Model file for the job. Use its own axes, mm. Round coordinates to 2 decimals unless told otherwise and drop trailing zeros. Order: outer loops, then holes, each group sorted by start corner. A loop starts at its lowest first (then second) coordinate and runs counter-clockwise, first axis right, second up. Notation, with made-up numbers: (51.25, -18.75) -> (81.25, -18.75) arc R30 cw to (81.25, 8.25) -> close; hole circle Ø7 at (-28.5, 0.25). An arc over 180 degrees is marked (long way). Put each result on its own line as item: value. Start each with the question number.
Q1. Cut at A-A, the plane x = 164.5. List the corners of the cut face in (y, z).
Q2. Cut at C-C, the plane y = 25. List the corners of the cut face in (x, z), and give its area (3 significant figures).
Q3. Pull direction Y, two halves, no side cores. Call faces 1 (the face through (162.502, 4.588, 150.493)), 2 (the face through (86, 68, 148)): released by +Y, released by -Y, zero draft, split by the parting line, or undercut.
Q4. Flat gauge pins, fed straight in: P1, Ø1.6, axis at x = 103.5, z = 148.5, coming from the +Y side; P2, Ø0.6, axis at x = 6, z = 149, coming from the -Y side; P3, Ø5, axis at x = 164.5, y = 129.5, coming from the -Z side. Where does each tip first touch, or does it go through?
Q5. Cut at D-D, the plane z = 149.2. List the corners of the cut face in (x, y).
Q6. Probe L1, parallel to Y at x = 164.5, z = 150.45; L2, parallel to X at y = 129.5, z = 150.7; L3, parallel to Y at x = 163, z = 150.4. List the from-to ranges inside material, lowest first.
Q7. Cut at B-B, the plane y = 4.5. List the corners of the cut face in (x, z), and give its area (3 significant figures).
from build123d import *

# Parameters (mm, degrees)
SKETCH008_W     = 175
SKETCH008_H     = 140
PAD002_DEPTH    = 3
PAD003_DEPTH    = 2
SKETCH010_R     = 2
POCKET006_DEPTH = 3.001
CHAMFER001_SIZE = 2
FILLET001_R     = 3


with BuildPart() as part:
    # Sketch008 → Pad002 (new body)
    with BuildSketch(Plane.XY):
        with Locations((84.5, 67)):
            Rectangle(SKETCH008_W, SKETCH008_H)
    extrude(amount=PAD002_DEPTH)

    # Sketch009 → Pad003 (join)
    with BuildSketch(Plane.XY):
        Polygon((0.5, 9.5), (0.5, 124.5), (9.5, 124.5), (9.5, 133.5), (159.5, 133.5), (159.5, 124.5), (168.5, 124.5), (168.5, 9.5), (159.5, 9.5), (159.5, 0.5), (9.5, 0.5), (9.5, 9.5), align=None)
    extrude(amount=-PAD003_DEPTH)

    # Sketch010 → Pocket006 (cut, through all)
    with BuildSketch(Plane.XY):
        with Locations((4.5, 4.5)):
            Circle(SKETCH010_R)
        with Locations((164.5, 129.5)):
            Circle(SKETCH010_R)
        with Locations((164.5, 4.5)):
            Circle(SKETCH010_R)
        with Locations((4.5, 129.5)):
            Circle(SKETCH010_R)
    extrude(amount=POCKET006_DEPTH, mode=Mode.SUBTRACT)

    # Chamfer001
    chamfer001_edges = [part.edges().sort_by_distance(p)[0] for p in [
        (2.5, 129.5, 3),
        (162.5, 129.5, 3),
        (162.5, 4.5, 3),
        (2.5, 4.5, 3),
    ]]
    chamfer(chamfer001_edges, length=CHAMFER001_SIZE)

    # Fillet001
    fillet001_edges = [part.edges().sort_by_distance(p)[0] for p in [
        (172, -3, 1.5),
        (172, 137, 1.5),
        (-3, -3, 1.5),
        (-3, 137, 1.5),
    ]]
    fillet(fillet001_edges, radius=FILLET001_R)


with BuildPart() as part_1:
    # Body placement: moved
    add(part.part.moved(Location((0, 0, 150))))


solid = part_1.part
Ans:
1. outline: (-3, 150) -> (2.5, 150) -> (2.5, 151) -> (0.5, 153) -> (-3, 153) -> close; (6.5, 150) -> (9.5, 150) -> (9.5, 148) -> (124.5, 148) -> (124.5, 150) -> (127.5, 150) -> (127.5, 151) -> (125.5, 153) -> (8.5, 153) -> (6.5, 151) -> close; (131.5, 150) -> (137, 150) -> (137, 153) -> (133.5, 153) -> (131.5, 151) -> close
2. outline: (-3, 150) -> (0.5, 150) -> (0.5, 148) -> (168.5, 148) -> (168.5, 150) -> (172, 150) -> (172, 153) -> (-3, 153) -> close
2. area: 861 mm^2
3. face 1: undercut
3. face 2: zero draft
4. P1: stops at y = 133.5
4. P2: stops at y = 9.5
4. P3: stops at z = 150
5. outline: (0.5, 9.5) -> (9.5, 9.5) -> (9.5, 0.5) -> (159.5, 0.5) -> (159.5, 9.5) -> (168.5, 9.5) -> (168.5, 124.5) -> (159.5, 124.5) -> (159.5, 133.5) -> (9.5, 133.5) -> (9.5, 124.5) -> (0.5, 124.5) -> close
6. L1: y = -3 to 2.5, 6.5 to 127.5, 131.5 to 137
6. L2: x = -3 to 2.5, 6.5 to 162.5, 166.5 to 172
6. L3: y = -3 to 3.18, 5.82 to 128.18, 130.82 to 137
7. outline: (-3, 150) -> (2.5, 150) -> (2.5, 151) -> (0.5, 153) -> (-3, 153) -> close; (6.5, 150) -> (9.5, 150) -> (9.5, 148) -> (159.5, 148) -> (159.5, 150) -> (162.5, 150) -> (162.5, 151) -> (160.5, 153) -> (8.5, 153) -> (6.5, 151) -> close; (166.5, 150) -> (172, 150) -> (172, 153) -> (168.5, 153) -> (166.5, 151) -> close
7. area: 793 mm^2
